Geometry: see drawing. Coordinates: mm, zero at the bounding-box minimum. A direction names the side the tool comes from. Give positions to 0.01 mm unless a question says otherwise; leave off trailing zeros. Write each loop counter-clockwise with the first axis right and the second up, starting at its lowest first coordinate (ties: lowest second). Pieces come first, ordered by that corner, then holes. Notation, with made-up numbers: M 1.25,14 L 8.25,14 A29 cw 8.25,52 Z; hole C 44.25,38 d6. An arc over 180 degrees is marked long. Use a Markdown table: item, result. Add a question column.
1) Section D-D on z = 68. Return the cut outline in (x, y), then the cut area to 3 significant figures.
2) Section A-A on x = 45.5. Return the cut outline in (y, z), then the cut area to 3 significant figures.
3) Pin query (flat end, axial travel): pin 1 (9.5 mm diameter, centred on y = 29, z = 15, fed in from -X); pin 2 (12 mm diameter, centred on x = 24, z = 38, fed in from +Y). Return the tip coordinate at first contact, or that it passes through.
4) Set-up query: the marked faces 1, 2 and 3. Return all of +Z, -Z, +X, -X, +Y, -Y with unobstructed straight access to the full face (end or side cutting, diameter ignored); none if empty.
5) Section B-B on z = 8. Return the cut outline in (x, y).
6) Line query: line 1 (Y direction, x = 6, z = 9); line 2 (Z direction, x = 37.5, y = 36); line 3 (X direction, y = 31.5, z = 22). Output: solid intervals per line, ascending.
7) Section C-C on y = 34. Return the cut outline in (x, z).
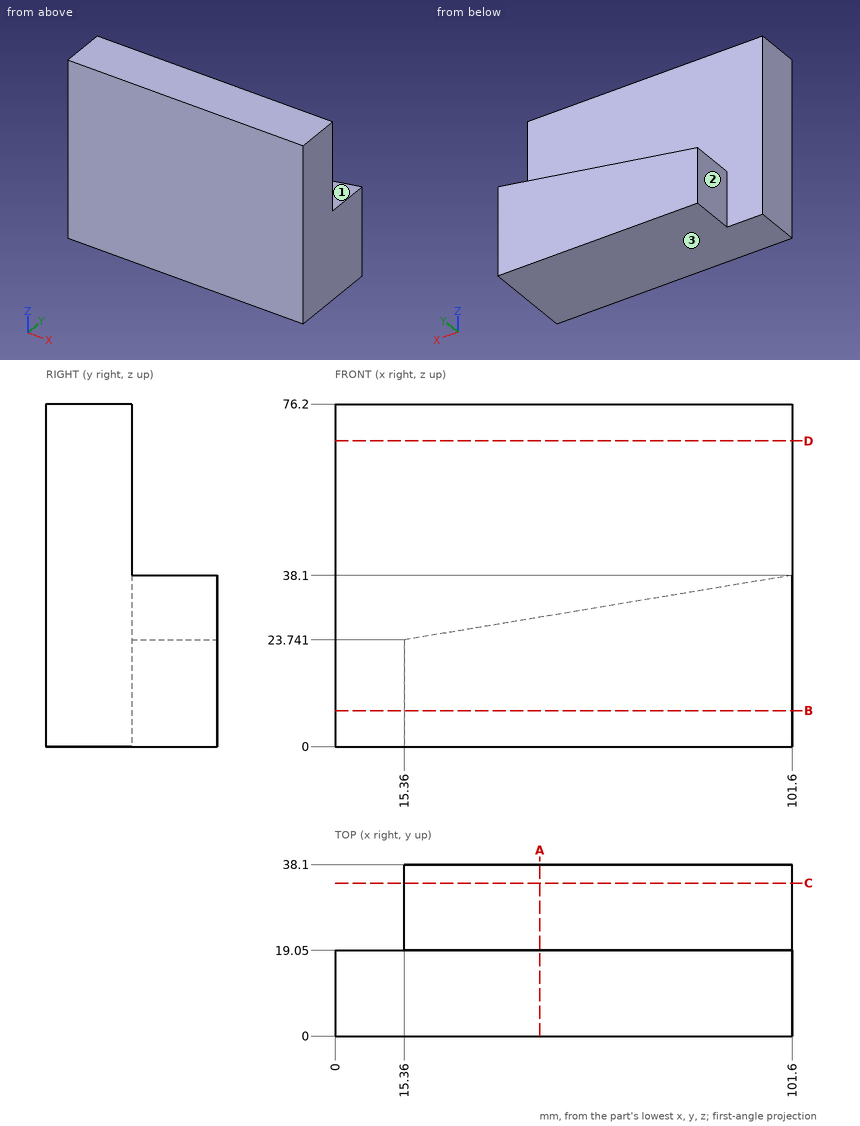
Found:
| question | item | result |
|---|---|---|
| 1 | outline | M 0,0 L 101.6,0 L 101.6,19.05 L 0,19.05 Z |
| 1 | area | 1,940 mm² |
| 2 | outline | M 0,0 L 38.1,0 L 38.1,28.76 L 19.05,28.76 L 19.05,76.2 L 0,76.2 Z |
| 2 | area | 2,000 mm² |
| 3 | pin 1 | x = 15.36 |
| 3 | pin 2 | y = 19.05 |
| 4 | face 1 | +Z, -X, +Y |
| 4 | face 2 | +Z, -Z, -X, +Y |
| 4 | face 3 | -Z, +X, -X, +Y, -Y |
| 5 | outline | M 0,0 L 101.6,0 L 101.6,38.1 L 15.36,38.1 L 15.36,19.05 L 0,19.05 Z |
| 6 | line 1 | 0 to 19.05 |
| 6 | line 2 | 0 to 27.43 |
| 6 | line 3 | 15.36 to 101.6 |
| 7 | outline | M 15.36,0 L 101.6,0 L 101.6,38.1 L 15.36,23.74 Z |
